```python
from build123d import *

# Parameters (mm, degrees)
F0_R     = 1.75
F0_R_2   = 4.85
F1_DEPTH = 2
F2_W     = 14
F2_H     = 2
F3_DEPTH = 12
F5_D     = 2.4


# Not quite as in the source:
# - a feature names something its author has since deleted; it is built from what else it names


with BuildPart() as f1:
    # F0 (on Front) → F1 (new body)
    with BuildSketch(Plane.XZ):
        with BuildLine():
            Line((9.2, 17.7), (-9.2, 17.7))
            ThreePointArc((-9.2, 17.7), (-14.8568542495, 15.3568542495), (-17.2, 9.7))
            Line((-17.2, 9.7), (-17.2, -15.7))
            Line((-17.2, -15.7), (17.2, -15.7))
            Line((17.2, -15.7), (17.2, 9.7))
            ThreePointArc((17.2, 9.7), (14.8568542495, 15.3568542495), (9.2, 17.7))
        make_face()
        with Locations((-0.1129766364, -11.55)):
            Circle(F0_R, mode=Mode.SUBTRACT)
        with Locations((-8.1, -8.1)):
            Circle(F0_R_2, mode=Mode.SUBTRACT)
        with Locations((-11.55, 0)):
            Circle(F0_R, mode=Mode.SUBTRACT)
        with Locations((8.1, -8.1)):
            Circle(F0_R_2, mode=Mode.SUBTRACT)
        with Locations((11.55, 0)):
            Circle(F0_R, mode=Mode.SUBTRACT)
        with Locations((-8.1, 8.1)):
            Circle(F0_R_2, mode=Mode.SUBTRACT)
        with Locations((-0.1129766364, 11.55)):
            Circle(F0_R, mode=Mode.SUBTRACT)
        with Locations((8.1, 8.1)):
            Circle(F0_R_2, mode=Mode.SUBTRACT)
    extrude(amount=F1_DEPTH)

    # F2 (on face) → F3 (join)
    with BuildSketch(Plane.XZ.offset(2)):
        with Locations((-10.2, -14.7)):
            Rectangle(F2_W, F2_H)
        with Locations((10.2, -14.7)):
            Rectangle(F2_W, F2_H)
    extrude(amount=F3_DEPTH)

    # F5 (through all)
    with Locations(Plane(origin=(0, 0, -15.7), x_dir=(1, 0, 0), z_dir=(0, 0, -1))):
        with Locations((-15, 11), (-15, 5), (15, 11), (15, 5)):
            Hole(F5_D / 2)


solid = f1.part
```
Geometry check sheet. Reference: the model listing, model coordinates, mm. A direction names the side the tool comes from. Round coordinates to 2 decimals unless told otherwise and drop trailing zeros. Write each loop counter-clockwise with the first axis right and the second up, starting at its lowest first coordinate (ties: lowest second). Pieces come first, ordered by that corner, then holes. Notation, with made-up numbers: (2.5, -9.75) -> (27.5, -9.75) arc R11 ccw to (27.5, 8.25) -> close; hole circle Ø9 at (-18.75, 55.25). An arc over 180 degrees is marked (long way). Put each result on its own line as item: value.
1) Release check for a two-part mould opening along X. For faces 1 (the face through (-10, -8, -13.7)), 2 (the face through (-3.2, -8, -15)), 3 (the face through (17.2, -1.8, -6.8)) record: pulls with the +X half, pulls with the -X half, needs draft (parallel to the pull), parting line crosses it, or undercut.
Recorded:
face 1: needs draft
face 2: undercut
face 3: pulls with the +X half
2) Cross-section at C-C, the plane y = -12.75. Enter the section's corners in (x, z), plus the area to 3 significant figures.
Recorded:
outline: (-17.2, -15.7) -> (-3.2, -15.7) -> (-3.2, -13.7) -> (-17.2, -13.7) -> close; (3.2, -15.7) -> (17.2, -15.7) -> (17.2, -13.7) -> (3.2, -13.7) -> close
area: 56.0 mm2
3) Access from +Z, -Z, +X, -X, +Y, -Y to the whole of each face (thin tool, end or side, straight path). Record for faces 4 (the face through (-4, -7, -15.7)), 5 (the face through (3.2, -8, -15)).
Recorded:
face 4: -Z, +X, -X, +Y, -Y
face 5: +Z, -Z, -Y
4) Cross-section at A-A, the plane z = 0. Enter the section's corners in (x, y).
Recorded:
outline: (-17.2, -2) -> (-13.3, -2) -> (-13.3, 0) -> (-17.2, 0) -> close; (-9.8, -2) -> (9.8, -2) -> (9.8, 0) -> (-9.8, 0) -> close; (13.3, -2) -> (17.2, -2) -> (17.2, 0) -> (13.3, 0) -> close
5) Thickness scan on probe 1 along Z at (x, y) = (8.1, -1.35); probe 2 along X at (y, z) = (-11, -15.1); probe 3 along X at (y, z) = (-12.75, -14). Record the ranges inside material, lowest first. Write a range as from..to.
Recorded:
probe 1: z = -15.7..-12.95, -3.25..3.25, 12.95..17.7
probe 2: x = -17.2..-16.2, -13.8..-3.2, 3.2..13.8, 16.2..17.2
probe 3: x = -17.2..-3.2, 3.2..17.2
6) Cross-section at B-B, the plane x = -15. Enter the section's corners in (y, z), plus the area to 3 significant figures.
Recorded:
outline: (-14, -15.7) -> (-12.2, -15.7) -> (-12.2, -13.7) -> (-14, -13.7) -> close; (-9.8, -15.7) -> (-6.2, -15.7) -> (-6.2, -13.7) -> (-9.8, -13.7) -> close; (-3.8, -15.7) -> (0, -15.7) -> (0, 15.21) -> (-2, 15.21) -> (-2, -13.7) -> (-3.8, -13.7) -> close
area: 76.2 mm2
7) Cross-section at D-D, the plane y = -5. Enter the section's corners in (x, z).
Recorded:
outline: (-17.2, -15.7) -> (-16.2, -15.7) -> (-16.2, -13.7) -> (-17.2, -13.7) -> close; (-13.8, -15.7) -> (-3.2, -15.7) -> (-3.2, -13.7) -> (-13.8, -13.7) -> close; (3.2, -15.7) -> (13.8, -15.7) -> (13.8, -13.7) -> (3.2, -13.7) -> close; (16.2, -15.7) -> (17.2, -15.7) -> (17.2, -13.7) -> (16.2, -13.7) -> close
8) Depth check by flat-ended pin: P1, Ø2, axis at x = -0.11, z = 11.55, coming from the +Y side; P2, Ø3, axis at x = -13.5, y = -12, coming from the +Z side. Enter the tip coordinate at first touch or a pass-through.
Recorded:
P1: passes through
P2: stops at z = -13.7
